Geometry check sheet. Reference: the model listing, model coordinates, mm. Face numbers are marked on the shaded views. A direction names the side the tool comes from. Give positions to 0.01 mm unless a question says otherwise; leave off trailing zeros. Write each loop counter-clockwise with the first axis right and the second up, starting at its lowest first coordinate (ties: lowest second). Pieces come first, ordered by that corner, then holes. Notation, with made-up numbers: (23, 24.5) - (54, 24.5) arc R8 cw to (54, 35.5) - close; hole circle Ø11 at (-22.75, 5). An arc over 180 degrees is marked (long way). Use a Markdown table: item, result.
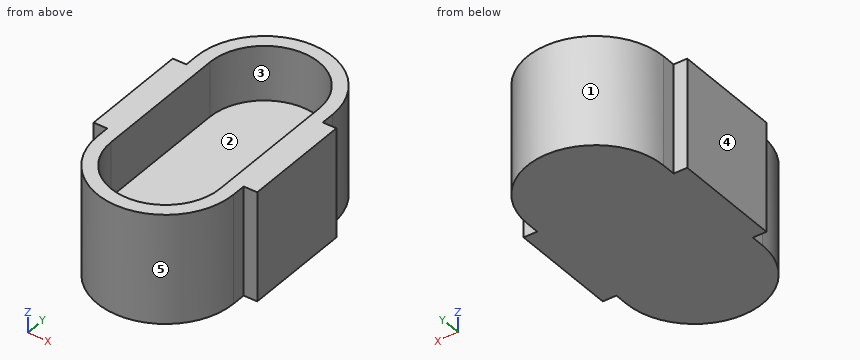
```python
from build123d import *

# Parameters (mm, degrees)
F1_DEPTH = 80
F2_DEPTH = 40
F0_W     = 10
F0_H     = 80
F3_DEPTH = 80


with BuildPart() as f1:
    # F0 (on Top) → F1 (new body)
    with BuildSketch(Plane.XY):
        with BuildLine():
            ThreePointArc((50, 50), (0, 100), (-50, 50))
            Line((-50, 50), (-50, 40))
            Line((-50, 40), (-50, -40))
            Line((-50, -40), (-50, -50))
            ThreePointArc((-50, -50), (0, -100), (50, -50))
            Line((50, -50), (50, -40))
            Line((50, -40), (50, 40))
            Line((50, 40), (50, 50))
        make_face()
        with BuildLine():
            Line((-40, -50), (-40, 50))
            ThreePointArc((-40, 50), (0, 90), (40, 50))
            Line((40, 50), (40, -50))
            ThreePointArc((40, -50), (0, -90), (-40, -50))
        make_face(mode=Mode.SUBTRACT)
    extrude(amount=F1_DEPTH)

    # F0 (on Top) → F2 (join)
    with BuildSketch(Plane.XY):
        with BuildLine():
            ThreePointArc((40, 50), (0, 90), (-40, 50))
            Line((-40, 50), (-40, -50))
            ThreePointArc((-40, -50), (0, -90), (40, -50))
            Line((40, -50), (40, 50))
        make_face()
    extrude(amount=F2_DEPTH)

    # F0 (on Top) → F3 (join)
    with BuildSketch(Plane.XY):
        with Locations((55, 0)):
            Rectangle(F0_W, F0_H)
        with Locations((-55, 0)):
            Rectangle(F0_W, F0_H)
    extrude(amount=F3_DEPTH)


solid = f1.part
```
1) Section check A-A on x = 0. Record the boundary of the cut face in (y, z), then the cut area to 3 significant figures.
Working result:
| item | result |
|---|---|
| outline | (-100, 0) - (100, 0) - (100, 80) - (90, 80) - (90, 40) - (-90, 40) - (-90, 80) - (-100, 80) - close |
| area | 8,800 mm² |
2) Section check B-B on z = 66. Record the boundary of the cut face in (x, y), then the cut area to 3 significant figures.
Working result:
| item | result |
|---|---|
| outline | (-60, -40) - (-50, -40) - (-50, -50) arc R50 ccw to (50, -50) - (50, -40) - (60, -40) - (60, 40) - (50, 40) - (50, 50) arc R50 ccw to (-50, 50) - (-50, 40) - (-60, 40) - close; hole (-40, -50) arc R40 ccw to (40, -50) - (40, 50) arc R40 ccw to (-40, 50) - close |
| area | 6,430 mm² |
3) Section check C-C on z = 20.5. Record the boundary of the cut face in (x, y).
Working result:
| item | result |
|---|---|
| outline | (-60, -40) - (-50, -40) - (-50, -50) arc R50 ccw to (50, -50) - (50, -40) - (60, -40) - (60, 40) - (50, 40) - (50, 50) arc R50 ccw to (-50, 50) - (-50, 40) - (-60, 40) - close |
4) Section check D-D on y = -80.5. Record the boundary of the cut face in (x, z), then the cut area to 3 significant figures.
Working result:
| item | result |
|---|---|
| outline | (-39.62, 0) - (39.62, 0) - (39.62, 80) - (25.88, 80) - (25.88, 40) - (-25.88, 40) - (-25.88, 80) - (-39.62, 80) - close |
| area | 4,270 mm² |
5) Depth check by flat-ended pin: P1, Ø5, axis at y = -44.5, z = 28, coming from the +X side; P2, Ø3, axis at x = -53.5, z = 34.5, coming from the -Y side; P3, Ø5, axis at x = 10, z = 8, coming from the -Y side. Enter the tip coordinate at first touch or a pass-through.
Working result:
| item | result |
|---|---|
| P1 | stops at x = 50 |
| P2 | stops at y = -40 |
| P3 | stops at y = -99.43 |
6) Set-up check for the marked faces 1 and 2: record each of +Z, -Z, +X, -X, +Y, -Y from which the full face is reachable in a straight line by a thin tool's end or side.
Working result:
| item | result |
|---|---|
| face 1 | +Z, -Z, +Y |
| face 2 | +Z |
7) Mould release check, pull along X, two halves, no side actions. Record for the marked faces 3, 4 and 5: pulls with the +X half, pulls with the -X half, needs draft (parallel to the pull), parting line crosses it, or undercut.
Working result:
| item | result |
|---|---|
| face 3 | undercut |
| face 4 | pulls with the -X half |
| face 5 | parting line crosses it |
8) Material ranges on L1, parallel to X at y = -1.5, z = 41.5; L2, parallel to Y at x = 0, z = 41; L3, parallel to Z at x = -29.5, y = -50, recorded low to high. Write a range as from..to.
Working result:
| item | result |
|---|---|
| L1 | x = -60..-40, 40..60 |
| L2 | y = -100..-90, 90..100 |
| L3 | z = 0..40 |
